Model file for the job. Use its own axes, mm. A direction names the side the tool comes from. Coordinates: 2 decimals unless noted, no trailing zeros. Write each loop counter-clockwise with the first axis right and the second up, starting at its lowest first coordinate (ties: lowest second). Pieces come first, ordered by that corner, then holes. Notation, with made-up numbers: M 18,15 L 67,15 A27 cw 67,35 Z; hole C -32.5,-29 d5. An arc over 180 degrees is marked long. Answer in a Markdown table with one row per item. Add a question column.
```python
from build123d import *

# Parameters (mm, degrees)
SZKIC1_W                    = 3
SZKIC1_H                    = 13
DODANIE_WYCI_GNI_CIE2_DEPTH = 13
SZKIC3_W                    = 6.769810996
SZKIC3_H                    = 13
DODANIE_WYCI_GNI_CIE3_DEPTH = 2
SZKIC4_R                    = 10
DODANIE_WYCI_GNI_CIE4_DEPTH = 3
SFAZOWANIE1_SIZE            = 0.25
SFAZOWANIE2_SIZE            = 0.25
ZAOKR_GLENIE2_R             = 5
SZKIC5_W                    = 2
SZKIC5_H                    = 11
DODANIE_WYCI_GNI_CIE5_DEPTH = 6
SZKIC8_W                    = 1
SZKIC8_H                    = 4
WYTNIJ_WYCI_GNI_CIE1_DEPTH  = 6


with BuildPart() as part:
    # Szkic1 → Dodanie-wyciągnięcie2 (new body)
    with BuildSketch(Plane(origin=(0, 0, 0), x_dir=(1, 0, 0), z_dir=(0, 1, 0))):
        Rectangle(SZKIC1_W, SZKIC1_H)
    extrude(amount=DODANIE_WYCI_GNI_CIE2_DEPTH)

    # Szkic3 → Dodanie-wyciągnięcie3 (add)
    with BuildSketch(Plane(origin=(1.5, 0, 0), x_dir=(0, 0, -1), z_dir=(1, 0, 0))):
        with Locations((0, 6.5)):
            Rectangle(SZKIC3_W, SZKIC3_H)
    extrude(amount=DODANIE_WYCI_GNI_CIE3_DEPTH)

    # Szkic4 → Dodanie-wyciągnięcie4 (add)
    with BuildSketch(Plane(origin=(3.5, 0, 0), x_dir=(0, 0, -1), z_dir=(1, 0, 0))):
        with Locations((0, 6.5)):
            Circle(SZKIC4_R)
    extrude(amount=DODANIE_WYCI_GNI_CIE4_DEPTH)

    # Sfazowanie1
    sfazowanie1_edges = [part.edges().sort_by_distance(p)[0] for p in [
        (6.5, 6.5, 10),
    ]]
    chamfer(sfazowanie1_edges, length=SFAZOWANIE1_SIZE)

    # Sfazowanie2
    sfazowanie2_edges = [part.edges().sort_by_distance(p)[0] for p in [
        (3.5, 6.5, 10),
    ]]
    chamfer(sfazowanie2_edges, length=SFAZOWANIE2_SIZE)

    # Zaokrąglenie2
    # the kernel refuses this fillet: 5 mm, written as the material it takes off along each edge
    with BuildSketch(Plane(origin=(6.5, 6.5, 0), x_dir=(0, 0, -1), z_dir=(0, -1, 0))) as zaokr_glenie2_piece_1:
        with BuildLine():
            CenterArc((8.4387505, -5), ZAOKR_GLENIE2_R, 71.805127661, 18.194872339)
            Line((8.4387505, 0), (8.4387505, 0.1))
            Line((8.4387505, 0.1), (9.75, 0.1))
            Line((9.75, 0.1), (9.820710678, 0.070710678))
            ThreePointArc((9.820710678, 0.070710678), (9.945710678, -0.054289322), (10.03122499, -0.155))
            Line((10.03122499, -0.155), (10, -0.25))
        make_face()
    revolve(axis=Axis((6.5, 6.5, 0), (1, 0, 0)), mode=Mode.SUBTRACT)

    # Szkic5 → Dodanie-wyciągnięcie5 (add)
    with BuildSketch(Plane.ZY.offset(1.5)):
        with Locations((0, 6.5)):
            Rectangle(SZKIC5_W, SZKIC5_H)
    extrude(amount=DODANIE_WYCI_GNI_CIE5_DEPTH)

    # Szkic8 → Wytnij-wyciągnięcie1 (cut)
    with BuildSketch(Plane(origin=(0, 0, -1), x_dir=(-1, 0, 0), z_dir=(0, 0, -1))):
        with Locations((5, 6.5)):
            Rectangle(SZKIC8_W, SZKIC8_H)
    extrude(amount=-WYTNIJ_WYCI_GNI_CIE1_DEPTH, mode=Mode.SUBTRACT)


solid = part.part
```
1) Slice it at C-C (x = 5.75). Give the cut face in (y, z).
2) Slice it at B-B (y = 6.5). Give the cut face in (x, z).
3) Which spindle directions (+Z, -Z, +X, -X, +Y, -Y) get a long thin tool onto all of the face, cutting with end or side? Do faces 5 (the face through (-5, 4.5, 0)), 6 (the face through (2, 6, 3.385)), 7 (the face through (-4, 1, 0)), 8 (the face through (-4, 6, 1)). Say none if no direction does.
4) Slice it at A-A (z = 0). Give the cut face in (x, y), then the cut area to 3 significant figures.
5) Two-plate mould, pull along X, no slides. Class faces 1 (the face through (-4.5, 6, 0)), 2 (the face through (2, 6, -3.385)), 3 (the face through (0, 6, 6.5)), 4 (the face through (6.5, 7, 0)): released by +X, released by -X, zero draft, split by the parting line, or undercut.
6) Drill centre lines: probe 1 along X at (y, z) = (1, -5.5); probe 2 along Z at (x, y) = (-6, 8.5); probe 3 along X at (y, z) = (11.5, 6.75). Where is each one in solid material? Low to high.
7) Slice it at D-D (x = -3.5). Give the cut face in (y, z), then the cut area to 3 significant figures.
8) Flat gauge pins, fed straight in: pin 1 Ø1.1 at (x, z) = (-5, -0.5) entering from -Y; pin 2 Ø5 at (x, y) = (-5, 14) entering from -Z; pin 3 Ø6.5 at (x, y) = (-4.5, 9) entering from +Z. Where does each tip first touch, or does it go through?
Ans:
| question | item | result |
|---|---|---|
| 1 | outline | C 6.5,0 d20 |
| 2 | outline | M -7.5,-1 L -5.5,-1 L -5.5,1 L -7.5,1 Z; M -4.5,-1 L -1.5,-1 L -1.5,-6.5 L 1.5,-6.5 L 1.5,-3.38 L 3.5,-3.38 L 3.5,-9.75 L 3.75,-10 L 6.25,-10 A5 ccw 6.5,-8.44 L 6.5,8.44 A5 ccw 6.25,10 L 3.75,10 L 3.5,9.75 L 3.5,3.38 L 1.5,3.38 L 1.5,6.5 L -1.5,6.5 L -1.5,1 L -4.5,1 Z |
| 3 | face 5 | +Z, -Z |
| 3 | face 6 | +Z, +Y, -Y |
| 3 | face 7 | +Z, -Z, -X, -Y |
| 3 | face 8 | +Z, -X, +Y, -Y |
| 4 | outline | M -7.5,1 L -1.5,1 L -1.5,0 L 3.5,0 L 3.5,-3.25 L 3.75,-3.5 L 6.25,-3.5 A5 ccw 6.5,-1.94 L 6.5,14.94 A5 ccw 6.25,16.5 L 3.75,16.5 L 3.5,16.25 L 3.5,13 L -1.5,13 L -1.5,12 L -7.5,12 Z; hole M -5.5,4.5 L -4.5,4.5 L -4.5,8.5 L -5.5,8.5 Z |
| 4 | area | 187 mm2 |
| 5 | face 1 | undercut |
| 5 | face 2 | undercut |
| 5 | face 3 | zero draft |
| 5 | face 4 | released by +X |
| 6 | probe 1 | x = -1.5 to 1.5, 3.5 to 6.5 |
| 6 | probe 2 | z = -1 to 1 |
| 6 | probe 3 | x = 3.5 to 6.5 |
| 7 | outline | M 1,-1 L 12,-1 L 12,1 L 1,1 Z |
| 7 | area | 22.0 mm2 |
| 8 | pin 1 | stops at y = 1 |
| 8 | pin 2 | stops at z = -1 |
| 8 | pin 3 | stops at z = 6.5 |
